from build123d import *

# Parameters (mm, degrees)
BOSS_EXTRUDE1_DEPTH     = 62
SKETCH2_R               = 18
BOSS_EXTRUDE2_DEPTH     = 2
SKETCH3_R               = 16
CUT_EXTRUDE1_DEPTH      = 74.391075752
CUT_EXTRUDE2_DEPTH      = 2
SKETCH5_R               = 3.5
CUT_EXTRUDE3_DEPTH      = 74.391075752
SKETCH6_W               = 48
SKETCH6_H               = 3
LPATTERN1_COUNT         = 9
LPATTERN1_PITCH         = 6
MIRROR1_COPY_1_SKETCH_W = 48
MIRROR1_COPY_1_SKETCH_H = 3
MIRROR1_COPY_2_SKETCH_W = 48
MIRROR1_COPY_2_SKETCH_H = 3
MIRROR1_COPY_3_SKETCH_W = 48
MIRROR1_COPY_3_SKETCH_H = 3
MIRROR1_COPY_4_SKETCH_W = 48
MIRROR1_COPY_4_SKETCH_H = 3
MIRROR1_COPY_5_SKETCH_W = 48
MIRROR1_COPY_5_SKETCH_H = 3
MIRROR1_COPY_6_SKETCH_W = 48
MIRROR1_COPY_6_SKETCH_H = 3
MIRROR1_COPY_7_SKETCH_W = 48
MIRROR1_COPY_7_SKETCH_H = 3
MIRROR1_COPY_8_SKETCH_W = 48
MIRROR1_COPY_8_SKETCH_H = 3
SKETCH8_W               = 48
SKETCH8_H               = 3
LPATTERN2_COUNT         = 9
LPATTERN2_PITCH         = 6


with BuildPart() as part:
    # Sketch1 → Boss-Extrude1 (new body)
    with BuildSketch(Plane(origin=(0, 0, 0), x_dir=(1, 0, 0), z_dir=(0, 1, 0))):
        with BuildLine():
            Line((-23, 22.5), (17, 22.5))
            ThreePointArc((17, 22.5), (20.535533906, 21.035533906), (22, 17.5))
            Line((22, 17.5), (22, -17.5))
            ThreePointArc((22, -17.5), (20.535533906, -21.035533906), (17, -22.5))
            Line((17, -22.5), (-23, -22.5))
            ThreePointArc((-23, -22.5), (-26.535533906, -21.035533906), (-28, -17.5))
            Line((-28, -17.5), (-28, 17.5))
            ThreePointArc((-28, 17.5), (-26.535533906, 21.035533906), (-23, 22.5))
        make_face()
    extrude(amount=BOSS_EXTRUDE1_DEPTH)

    # Sketch2 → Boss-Extrude2 (add)
    with BuildSketch(Plane(origin=(0, 62, 0), x_dir=(1, 0, 0), z_dir=(0, 1, 0))):
        with Locations(Location((0, 0, 0), (0, 0, 270))):
            Circle(SKETCH2_R)
    extrude(amount=BOSS_EXTRUDE2_DEPTH)

    # Sketch3 → Cut-Extrude1 (cut, through all)
    with BuildSketch(Plane(origin=(0, 64, 0), x_dir=(1, 0, 0), z_dir=(0, 1, 0))):
        with Locations(Location((0, 0, 0), (0, 0, 270))):
            Circle(SKETCH3_R)
    extrude(amount=-CUT_EXTRUDE1_DEPTH, mode=Mode.SUBTRACT)

    # Sketch4 → Cut-Extrude2 (cut)
    with BuildSketch(Plane.XZ):
        with BuildLine():
            Line((-22.61, 2), (-8.699965398, 2))
            Line((-8.699965398, 2), (-8.699965398, -2))
            Line((-8.699965398, -2), (-22.61, -2))
            ThreePointArc((-22.61, -2), (-24.61, 0), (-22.61, 2))
        make_face()
    extrude(amount=-CUT_EXTRUDE2_DEPTH, mode=Mode.SUBTRACT)

    # Sketch5 → Cut-Extrude3 (cut, through all)
    with BuildSketch(Plane.XZ):
        with Locations(Location((16.263455967, 16.263455967, 0), (0, 0, 270))):
            Circle(SKETCH5_R)
        with Locations(Location((16.263455967, -16.263455967, 0), (0, 0, 270))):
            Circle(SKETCH5_R)
        with Locations(Location((-16.263455967, -16.263455967, 0), (0, 0, 270))):
            Circle(SKETCH5_R)
        with Locations(Location((-16.263455967, 16.263455967, 0), (0, 0, 270))):
            Circle(SKETCH5_R)
    extrude(amount=-CUT_EXTRUDE3_DEPTH, mode=Mode.SUBTRACT)

    # Sketch6 → Cut-Revolve1 (revolve, cut)
    with BuildSketch(Plane(origin=(-3, 0, 0), x_dir=(0, 0, -1), z_dir=(1, 0, 0))):
        with Locations((-42.5, 5.5)):
            Rectangle(SKETCH6_W, SKETCH6_H)
    cut_revolve1 = revolve(axis=Axis((-3, 7, 66.5), (0, -1, 0)), mode=Mode.SUBTRACT)

    # LPattern1: Cut-Revolve1 ×9
    with Locations(*[(0, i * LPATTERN1_PITCH, 0) for i in range(1, LPATTERN1_COUNT)]):
        add(cut_revolve1, mode=Mode.SUBTRACT)

    # Mirror1: Cut-Revolve1 across plane
    add(cut_revolve1.mirror(Plane.XY), mode=Mode.SUBTRACT)

    # Mirror1 copy 1 sketch → Mirror1 copy 1 (revolve, cut)
    with BuildSketch(Plane(origin=(-3, 6, 0), x_dir=(0, 0, 1), z_dir=(1, 0, 0))):
        with Locations((-42.5, -5.5)):
            Rectangle(MIRROR1_COPY_1_SKETCH_W, MIRROR1_COPY_1_SKETCH_H)
    revolve(axis=Axis((-3, 13, -66.5), (0, 1, 0)), mode=Mode.SUBTRACT)

    # Mirror1 copy 2 sketch → Mirror1 copy 2 (revolve, cut)
    with BuildSketch(Plane(origin=(-3, 12, 0), x_dir=(0, 0, 1), z_dir=(1, 0, 0))):
        with Locations((-42.5, -5.5)):
            Rectangle(MIRROR1_COPY_2_SKETCH_W, MIRROR1_COPY_2_SKETCH_H)
    revolve(axis=Axis((-3, 19, -66.5), (0, 1, 0)), mode=Mode.SUBTRACT)

    # Mirror1 copy 3 sketch → Mirror1 copy 3 (revolve, cut)
    with BuildSketch(Plane(origin=(-3, 18, 0), x_dir=(0, 0, 1), z_dir=(1, 0, 0))):
        with Locations((-42.5, -5.5)):
            Rectangle(MIRROR1_COPY_3_SKETCH_W, MIRROR1_COPY_3_SKETCH_H)
    revolve(axis=Axis((-3, 25, -66.5), (0, 1, 0)), mode=Mode.SUBTRACT)

    # Mirror1 copy 4 sketch → Mirror1 copy 4 (revolve, cut)
    with BuildSketch(Plane(origin=(-3, 24, 0), x_dir=(0, 0, 1), z_dir=(1, 0, 0))):
        with Locations((-42.5, -5.5)):
            Rectangle(MIRROR1_COPY_4_SKETCH_W, MIRROR1_COPY_4_SKETCH_H)
    revolve(axis=Axis((-3, 31, -66.5), (0, 1, 0)), mode=Mode.SUBTRACT)

    # Mirror1 copy 5 sketch → Mirror1 copy 5 (revolve, cut)
    with BuildSketch(Plane(origin=(-3, 30, 0), x_dir=(0, 0, 1), z_dir=(1, 0, 0))):
        with Locations((-42.5, -5.5)):
            Rectangle(MIRROR1_COPY_5_SKETCH_W, MIRROR1_COPY_5_SKETCH_H)
    revolve(axis=Axis((-3, 37, -66.5), (0, 1, 0)), mode=Mode.SUBTRACT)

    # Mirror1 copy 6 sketch → Mirror1 copy 6 (revolve, cut)
    with BuildSketch(Plane(origin=(-3, 36, 0), x_dir=(0, 0, 1), z_dir=(1, 0, 0))):
        with Locations((-42.5, -5.5)):
            Rectangle(MIRROR1_COPY_6_SKETCH_W, MIRROR1_COPY_6_SKETCH_H)
    revolve(axis=Axis((-3, 43, -66.5), (0, 1, 0)), mode=Mode.SUBTRACT)

    # Mirror1 copy 7 sketch → Mirror1 copy 7 (revolve, cut)
    with BuildSketch(Plane(origin=(-3, 42, 0), x_dir=(0, 0, 1), z_dir=(1, 0, 0))):
        with Locations((-42.5, -5.5)):
            Rectangle(MIRROR1_COPY_7_SKETCH_W, MIRROR1_COPY_7_SKETCH_H)
    revolve(axis=Axis((-3, 49, -66.5), (0, 1, 0)), mode=Mode.SUBTRACT)

    # Mirror1 copy 8 sketch → Mirror1 copy 8 (revolve, cut)
    with BuildSketch(Plane(origin=(-3, 48, 0), x_dir=(0, 0, 1), z_dir=(1, 0, 0))):
        with Locations((-42.5, -5.5)):
            Rectangle(MIRROR1_COPY_8_SKETCH_W, MIRROR1_COPY_8_SKETCH_H)
    revolve(axis=Axis((-3, 55, -66.5), (0, 1, 0)), mode=Mode.SUBTRACT)

    # Sketch8 → Cut-Revolve3 (revolve, cut)
    with BuildSketch(Plane.XY):
        with Locations((-48, 5.5)):
            Rectangle(SKETCH8_W, SKETCH8_H)
    cut_revolve3 = revolve(axis=Axis((-72, 7, 0), (0, -1, 0)), mode=Mode.SUBTRACT)

    # LPattern2: Cut-Revolve3 ×9
    with Locations(*[(0, i * LPATTERN2_PITCH, 0) for i in range(1, LPATTERN2_COUNT)]):
        add(cut_revolve3, mode=Mode.SUBTRACT)


solid = part.part
Source: CAD feature listing. Evaluate the final solid. Frame: model axes, mm. A direction names the side the tool comes from. Round coordinates to 2 decimals unless told otherwise and drop trailing zeros. Loops run counter-clockwise (first coordinate to the right, second up) from the corner with the lowest first, then second, coordinate; pieces in that order, holes last. Notation, with made-up numbers: M 74,43 L 91,43 A13 cw 91,54 Z; hole C 41,21 d3. An arc over 180 degrees is marked long. Return JSON: item names as keys, results as strings. Group by question number.
1. Section query D-D on y = 60. Output: boundary loops of the cut face in (x, z).
2. Material intervals for line 1 along X through (y, z) = (50.5, 16.5); line 2 along X through (y, z) = (5.5, -5); line 3 along X through (y, z) = (60.5, -11), sorted ascending. Write a range as from..to.
3. Reachability of faces 1 (the face through (-3, 43, 21)), 2 (the face through (-26, 37, 0)), 3 (the face through (-3, 40, -21)) from +Z, -Z, +X, -X, +Y, -Y: full face, straight path, thin tool, end or side. Return the list, or none.
4. Section query B-B on z = 15. State how many separate pieces and enclosed holes the cut face has, and give its area (3 significant figures).
5. Mould query, pull axis X, two halves, no side actions, for faces 4 (the face through (-3.3, 37.5, -22.5)), 5 (the face through (-3, 10, 21)), 6 (the face through (-28, 2, 0)), 7 (the face through (-3, 13, -21)). Classes: released by +X, released by -X, zero draft, split by the parting line, or undercut.
6. Pin query (flat end, axial travel): pin 1 (4.5 mm diameter, centred on x = -11, z = -20.5, fed in from +Y); pin 2 (5.5 mm diameter, centred on x = 16.26, z = 16.26, fed in from -Y). Return the tip coordinate at first contact, or that it passes through.
7. Section query A-A on y = 36. Output: boundary loops of the cut face in (x, z), and give its area (3 significant figures).
Checks:
{
 "1": {"outline": "M -28,-17.5 A5 ccw -23,-22.5 L 17,-22.5 A5 ccw 22,-17.5 L 22,17.5 A5 ccw 17,22.5 L -23,22.5 A5 ccw -28,17.5 Z; hole C -16.26,-16.26 d7; hole C -16.26,16.26 d7; hole C 0,0 d32; hole C 16.26,-16.26 d7; hole C 16.26,16.26 d7"},
 "2": {"line 1": "x = -28..-19.76, -12.77..12.77, 19.76..22", "line 2": "x = -24.26..-15.2, 15.2..22", "line 3": "x = -28..-11.62, 11.62..22"},
 "3": {"face 1": "+Z", "face 2": "-X", "face 3": "-Z"},
 "4": {"separate pieces": "4", "enclosed holes": "0", "area": "1,570 mm²"},
 "5": {"face 4": "zero draft", "face 5": "undercut", "face 6": "released by -X", "face 7": "undercut"},
 "6": {"pin 1": "stops at y = 62", "pin 2": "passes through"},
 "7": {"outline": "M -27.83,-18.79 A5 ccw -23,-22.5 L -22.18,-22.5 A48 cw 16.18,-22.5 L 17,-22.5 A5 ccw 22,-17.5 L 22,17.5 A5 ccw 17,22.5 L 16.18,22.5 A48 cw -22.18,22.5 L -23,22.5 A5 ccw -27.83,18.79 A48 cw Z; hole C -16.26,-16.26 d7; hole C -16.26,16.26 d7; hole C 0,0 d32; hole C 16.26,-16.26 d7; hole C 16.26,16.26 d7", "area": "961 mm²"}
}
